from build123d import *

# Parameters (mm, degrees)
SKETCH1_R           = 75
SKETCH1_R_2         = 62.6
SKETCH1_R_3         = 7.5
SKETCH1_R_4         = 1.7
BOSS_EXTRUDE1_DEPTH = 10
FILLET1_R           = 10
SKETCH2_R           = 75
SKETCH2_R_2         = 62.6
BOSS_EXTRUDE2_DEPTH = 15


with BuildPart() as part:
    # Sketch1 → Boss-Extrude1 (new body)
    # profile 1 of 5: a face of its own
    with BuildSketch(Plane(origin=(0, 0, 0), x_dir=(1, 0, 0), z_dir=(0, 1, 0))):
        Circle(SKETCH1_R)
        with Locations(Location((0, 0, 0), (0, 0, 270))):
            Circle(SKETCH1_R_2, mode=Mode.SUBTRACT)
    # profile 2 of 5: a face of its own
    with BuildSketch(Plane(origin=(0, 0, 0), x_dir=(1, 0, 0), z_dir=(0, 1, 0))):
        with Locations((0, 80)):
            Circle(SKETCH1_R_3)
        with Locations(Location((0, 80, 0), (0, 0, 270))):
            Circle(SKETCH1_R_4, mode=Mode.SUBTRACT)
    # profile 3 of 5: a face of its own
    with BuildSketch(Plane(origin=(0, 0, 0), x_dir=(1, 0, 0), z_dir=(0, 1, 0))):
        with Locations((79.975806452, 0.024193548)):
            Circle(SKETCH1_R_3)
        with Locations(Location((79.975806452, 0.024193548, 0), (0, 0, 270))):
            Circle(SKETCH1_R_4, mode=Mode.SUBTRACT)
    # profile 4 of 5: a face of its own
    with BuildSketch(Plane(origin=(0, 0, 0), x_dir=(1, 0, 0), z_dir=(0, 1, 0))):
        with Locations((0, -79.951612903)):
            Circle(SKETCH1_R_3)
        with Locations(Location((0, -79.951612903, 0), (0, 0, 270))):
            Circle(SKETCH1_R_4, mode=Mode.SUBTRACT)
    # profile 5 of 5: a face of its own
    with BuildSketch(Plane(origin=(0, 0, 0), x_dir=(1, 0, 0), z_dir=(0, 1, 0))):
        with Locations((-79.975806452, 0.024193548)):
            Circle(SKETCH1_R_3)
        with Locations(Location((-79.975806452, 0.024193548, 0), (0, 0, 270))):
            Circle(SKETCH1_R_4, mode=Mode.SUBTRACT)
    extrude(amount=BOSS_EXTRUDE1_DEPTH)

    # Fillet1
    fillet1_edges = [part.edges().sort_by_distance(p)[0] for p in [
        (-74.804759202, 5, 5.408142077),
        (-74.801473468, 5, -5.453399584),
        (5.452241155, 5, 74.801557914),
        (-5.452241155, 5, 74.801557914),
        (74.801473468, 5, -5.453399584),
        (74.804759202, 5, 5.408142077),
        (-5.409133759, 5, -74.8046875),
        (5.409133759, 5, -74.8046875),
    ]]
    fillet(fillet1_edges, radius=FILLET1_R)

    # Sketch2 → Boss-Extrude2 (add)
    with BuildSketch(Plane(origin=(0, 10, 0), x_dir=(1, 0, 0), z_dir=(0, 1, 0))):
        with Locations(Location((0, 0, 0), (0, 0, 78.327450214))):
            Circle(SKETCH2_R)
        with Locations(Location((0, 0, 0), (0, 0, 270))):
            Circle(SKETCH2_R_2, mode=Mode.SUBTRACT)
    extrude(amount=BOSS_EXTRUDE2_DEPTH)


solid = part.part
The model under review builds one solid part; all positions refer to its coordinate system, in mm. A direction names the side the tool comes from. Give positions to 0.01 mm unless a question says otherwise; leave off trailing zeros. Write each loop counter-clockwise with the first axis right and the second up, starting at its lowest first coordinate (ties: lowest second). Pieces come first, ordered by that corner, then holes.
1. For P1, Ø3, axis at y = 19.5, z = 15.5, coming from the +X side; P2, Ø3, axis at x = 0, z = -80, coming from the -Y side; P3, Ø5, axis at y = 7, z = -39, coming from the -X side; P4, Ø10, axis at x = -13, y = 9, coming from the -Z side, all flat-tipped, find the tip position at first contact; note any pin that passes through.
2. Tool access review of faces 4 (the flat face through (56, 25, 29)), 5 (the cylindrical face through (63.323, 9.547, -40.19)): name each direction out of +Z, -Z, +X, -X, +Y, -Y from which nothing blocks a thin tool from reaching the whole face with its end or side.
3. Wall thickness on L1, parallel to X at y = 9.75, z = 0; L2, parallel to Z at x = 22.5, y = 11.25; L3, parallel to Z at x = 34.5, y = 19: over which ranges is each line inside the solid? List them lowest first.
4. Add section C-C, the plane x = -69. Write out the cut boundary in (y, z), plus the area to 3 significant figures.
5. Add section A-A, the plane z = 4.5. Write out the cut boundary in (x, y), plus the area to 3 significant figures.
6. Add section B-B, the plane y = 23. Write out the cut boundary in (x, z), plus the area to 3 significant figures.
7. Draft analysis for pull direction Z (two halves, no side actions). For faces 1 (the flat face through (0, 10, -82)), 2 (the cylindrical face through (-87.474, 4.93, -0.172)), 3 (the cylindrical face through (62.067, 12.325, -8.149)), state which applies: +Z half, -Z half, draft (parallel to the pull), parting line (faces both ways), or undercut.
Worked answers:
1. P1: stops at x = 73.68
1. P2: passes through
1. P3: stops at x = -65.52
1. P4: stops at z = -79.32
2. face 4: +Z, -Z, +X, -X, +Y
2. face 5: +Y
3. L1: x = -87.48 to -81.68, -78.28 to -62.6, 62.6 to 78.28, 81.68 to 87.48
3. L2: z = -71.55 to -58.42, 58.42 to 71.55
3. L3: z = -66.59 to -52.24, 52.24 to 66.59
4. outline: (0, -29.39) - (25, -29.39) - (25, 29.39) - (0, 29.39) - close
4. area: 1,470 mm2
5. outline: (-85.96, 0) - (-62.44, 0) - (-62.44, 25) - (-74.86, 25) - (-74.86, 10) - (-85.96, 10) - close; (62.44, 0) - (85.96, 0) - (85.96, 10) - (74.86, 10) - (74.86, 25) - (62.44, 25) - close
5. area: 843 mm2
6. outline: circle Ø150 at (0, 0); hole circle Ø125.2 at (0, 0)
6. area: 5,360 mm2
7. face 1: draft
7. face 2: parting line
7. face 3: undercut
